Can you work these out from the model? Positions are in its coordinate system, mm. Face numbers are marked on the shaded views. Give positions to 0.01 mm unless a question says otherwise; leave off trailing zeros. Loops run counter-clockwise (first coordinate to the right, second up) from the corner with the lowest first, then second, coordinate; pieces in that order, holes last. Notation, with made-up numbers: (59.5, 30) -> (83.5, 30) arc R21 cw to (83.5, 40) -> close; hole circle Ø9 at (-24.75, 50). An arc over 180 degrees is marked (long way). One line per question, with ' | ' between items.
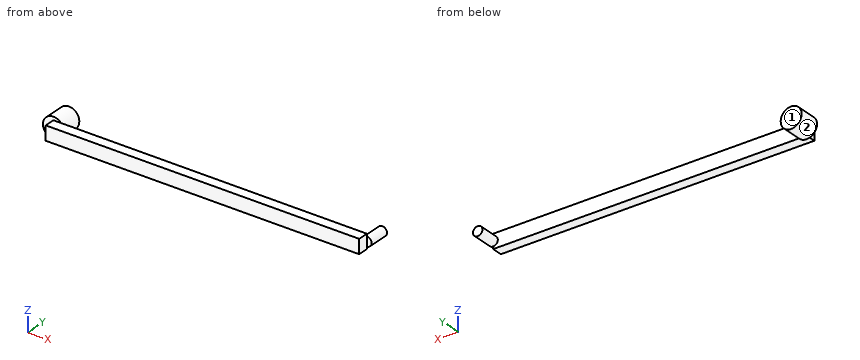
from build123d import *

# Parameters (mm, degrees)
SKETCH1_W           = 76.2
SKETCH1_H           = 3.45052473
BOSS_EXTRUDE1_DEPTH = 2.54
SKETCH2_R           = 2.54
BOSS_EXTRUDE2_DEPTH = 5.08
SKETCH3_R           = 1.143
BOSS_EXTRUDE3_DEPTH = 5.08


with BuildPart() as part:
    # Sketch1 → Boss-Extrude1 (new body)
    with BuildSketch(Plane(origin=(0, 0, 0), x_dir=(1, 0, 0), z_dir=(0, 1, 0))):
        Rectangle(SKETCH1_W, SKETCH1_H)
    extrude(amount=BOSS_EXTRUDE1_DEPTH)

    # Sketch2 → Boss-Extrude2 (add)
    with BuildSketch(Plane(origin=(0, 2.54, 0), x_dir=(1, 0, 0), z_dir=(0, 1, 0))):
        with Locations((-38.1, 0)):
            Circle(SKETCH2_R)
    extrude(amount=BOSS_EXTRUDE2_DEPTH)

    # Sketch3 → Boss-Extrude3 (add)
    with BuildSketch(Plane(origin=(0, 2.54, 0), x_dir=(1, 0, 0), z_dir=(0, 1, 0))):
        with Locations((38.1, 0)):
            Circle(SKETCH3_R)
    extrude(amount=BOSS_EXTRUDE3_DEPTH)


solid = part.part
Q1. For pin 1 Ø3 at (x, y) = (5, 1.5) entering from +Z; pin 2 Ø3 at (y, z) = (1, -0.5) entering from +X; pin 3 Ø0.9 at (x, z) = (39, 0) entering from -Y, each with a flat end and sliding along its axis, tell me the tip position at first contact or that it passes through.
Entries:
pin 1: z = 1.73 | pin 2: x = 38.1 | pin 3: y = 2.54
Q2. If I drill on probe 1 along X at (y, z) = (2.25, -0.5); probe 2 along Y at (x, z) = (6.5, 1.05); probe 3 along X at (y, z) = (6.25, -0.4), over which ranges is the centre line in solid material (lowest first)? Write a range as from..to.
Entries:
probe 1: -38.1..38.1 | probe 2: 0..2.54 | probe 3: -40.61..-35.59, 37.03..39.17
Q3. If we mould it in two halves opening along X, with no side actions, what happens to the marked faces 1 and 2? For each: pulls with the +X half, pulls with the -X half, needs draft (parallel to the pull), parting line crosses it, or undercut.
Entries:
face 1: needs draft | face 2: undercut
Q4. If we section it at B-B (x = -17.5): Write out the boundary of the cut face in (y, z), plus the area to 3 significant figures.
Entries:
outline: (0, -1.73) -> (2.54, -1.73) -> (2.54, 1.73) -> (0, 1.73) -> close | area: 8.76 mm²
Q5. If we section it at A-A (y = 6): Write out the boundary of the cut face in (x, z).
Entries:
outline: circle Ø5.08 at (-38.1, 0); circle Ø2.29 at (38.1, 0)
